from build123d import *

# Parameters (mm, degrees)
BOSS_EXTRUDE1_DEPTH = 25.4
SKETCH2_R           = 7.332348419
SKETCH2_R_2         = 4.7625
CUT_EXTRUDE1_DEPTH  = 7.9375
CUT_EXTRUDE2_START  = -7.9375
SKETCH3_R           = 7.332348419
SKETCH3_R_2         = 4.7625
CUT_EXTRUDE2_DEPTH  = 7.9375


with BuildPart() as part:
    # Sketch1 → Boss-Extrude1 (new, symmetric)
    with BuildSketch(Plane.XY):
        Polygon((3.684589596, -6.339332208), (7.332317533, 0.021282089), (3.647727937, 6.360614297), (-3.684589596, 6.339332208), (-7.332317533, -0.021282089), (-3.647727937, -6.360614297), align=None)
    extrude(amount=BOSS_EXTRUDE1_DEPTH, both=True)

    # Sketch2 → Cut-Extrude1 (cut)
    with BuildSketch(Plane.XY.offset(25.4)):
        Circle(SKETCH2_R)
        Circle(SKETCH2_R_2, mode=Mode.SUBTRACT)
    extrude(amount=-CUT_EXTRUDE1_DEPTH, mode=Mode.SUBTRACT)

    # Sketch3 → Cut-Extrude2 (cut)
    with BuildSketch(Plane(origin=(0, 0, -25.4), x_dir=(-1, 0, 0), z_dir=(0, 0, -1)).offset(CUT_EXTRUDE2_START)):
        Circle(SKETCH3_R)
        with Locations(Location((0, 0, 0), (0, 0, 180))):
            Circle(SKETCH3_R_2, mode=Mode.SUBTRACT)
    extrude(amount=CUT_EXTRUDE2_DEPTH, mode=Mode.SUBTRACT)


solid = part.part
Geometry: final body of the model. Coordinates: model frame, mm. A direction names the side the tool comes from. Give positions to 0.01 mm unless a question says otherwise; leave off trailing zeros. Loops run counter-clockwise (first coordinate to the right, second up) from the corner with the lowest first, then second, coordinate; pieces in that order, holes last. Notation, with made-up numbers: (-11, 57.5) -> (-2, 57.5) arc R30 ccw to (-2, 93.5) -> close; hole circle Ø2 at (43, -3.75). An arc over 180 degrees is marked (long way). Put each result on its own line as item: value.
1. Cut plane B-B (z = -1). Return the cut outline in (x, y).
Taken from the geometry:
outline: (-7.33, -0.02) -> (-3.65, -6.36) -> (3.68, -6.34) -> (7.33, 0.02) -> (3.65, 6.36) -> (-3.68, 6.34) -> close
2. Pin query (flat end, axial travel): P1, Ø1, axis at y = -1, z = 12.5, coming from the -X side; P2, Ø1.5, axis at y = 4.5, z = -5, coming from the +X side; P3, Ø6, axis at x = 3.5, z = 19, coming from the -Y side. Return the tip coordinate at first contact, or that it passes through.
Taken from the geometry:
P1: stops at x = -7.05
P2: stops at x = 5.17
P3: stops at y = -6.35
3. Set-up query: faces 1 (the cylindrical face through (-1.03, 4.65, -21.38)), 2 (the flat face through (0, 0, -25.4)), 3 (the cylindrical face through (-3.78, -2.9, 21.49)). Return all of +Z, -Z, +X, -X, +Y, -Y with unobstructed straight access to the full face (end or side cutting, diameter ignored); none if empty.
Taken from the geometry:
face 1: -Z
face 2: -Z, +X, -X, +Y, -Y
face 3: +Z
4. Cut plane A-A (y = -1.75). Return the cut outline in (x, z).
Taken from the geometry:
outline: (-6.33, -17.46) -> (-4.43, -17.46) -> (-4.43, -25.4) -> (4.43, -25.4) -> (4.43, -17.46) -> (6.32, -17.46) -> (6.32, 17.46) -> (4.43, 17.46) -> (4.43, 25.4) -> (-4.43, 25.4) -> (-4.43, 17.46) -> (-6.33, 17.46) -> close
5. Ray query, line 1 along Z through (x, y) = (1.5, -5); line 2 along Y through (x, z) = (3.5, -10); line 3 along Y through (x, z) = (-1, -2.5). Return the intervals inside material, ascending. Write a range as [from, to].
Taken from the geometry:
line 1: z = [-17.46, 17.46]
line 2: y = [-6.34, 6.36]
line 3: y = [-6.35, 6.35]
6. Cut plane C-C (x = 0). Return the cut outline in (y, z), plus the area to 3 significant figures.
Taken from the geometry:
outline: (-6.35, -17.46) -> (-4.76, -17.46) -> (-4.76, -25.4) -> (4.76, -25.4) -> (4.76, -17.46) -> (6.35, -17.46) -> (6.35, 17.46) -> (4.76, 17.46) -> (4.76, 25.4) -> (-4.76, 25.4) -> (-4.76, 17.46) -> (-6.35, 17.46) -> close
area: 595 mm2
